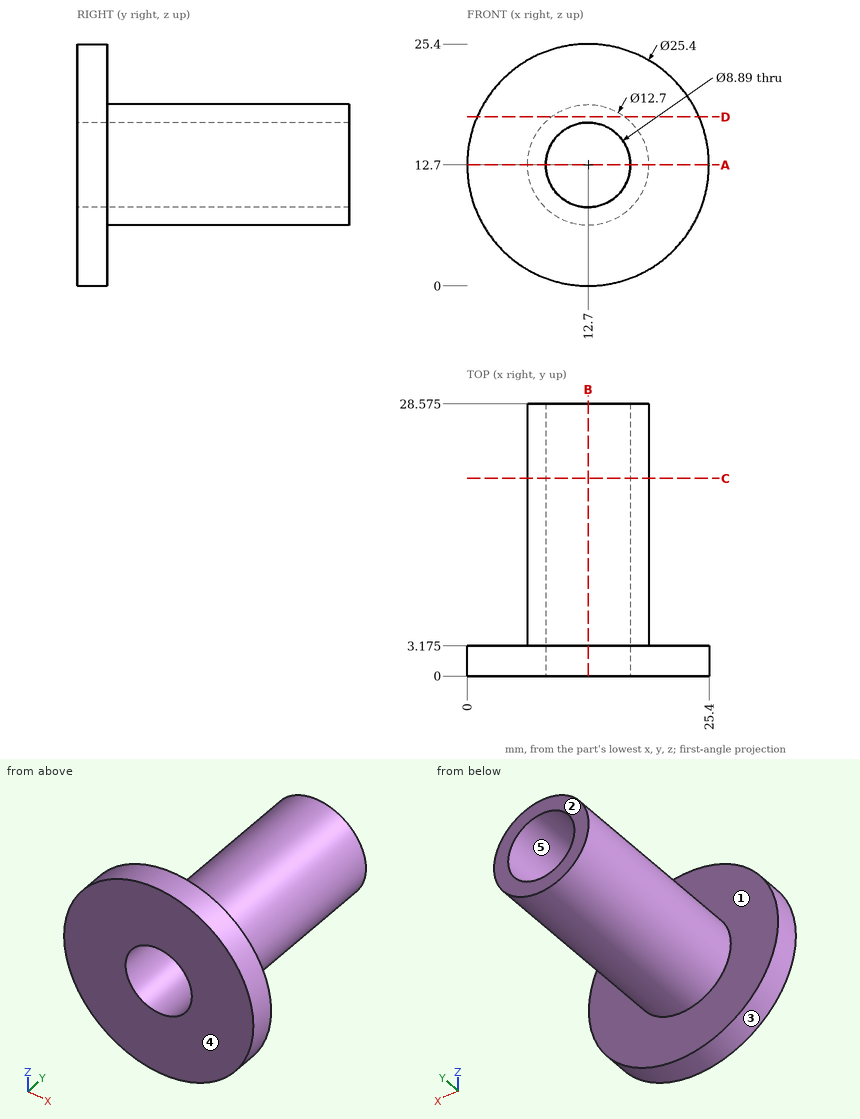
Print and shaded views of the part. All mm, measured from the part's lowest x, y and z. A direction names the side the tool comes from. Give positions to 0.01 mm unless a question says otherwise; leave off trailing zeros. Loops run counter-clockwise (first coordinate to the right, second up) from the corner with the lowest first, then second, coordinate; pieces in that order, holes last. Notation, with made-up numbers: (20.5, 1) -> (52.5, 1) arc R8 ccw to (52.5, 11) -> close; hole circle Ø9 at (-3.5, -9). An arc over 180 degrees is marked (long way). Answer in a Markdown table with one row per item.
Item 1: Tool access for the marked faces 1 and 2: list every direction of +Z, -Z, +X, -X, +Y, -Y with a clear straight run to the whole face (end or side of a thin tool).
Findings below:
| item | result |
|---|---|
| face 1 | +Y |
| face 2 | +Z, -Z, +X, -X, +Y |
Item 2: Flat gauge pins, fed straight in: P1, Ø10, axis at y = 20.5, z = 16, coming from the -X side; P2, Ø3, axis at x = 7.5, z = 20.5, coming from the +Y side (3 decimals); P3, Ø1.5, axis at x = 18.5, y = 16.5, coming from the -Z side. Where does each tip first touch, or does it go through?
Findings below:
| item | result |
|---|---|
| P1 | stops at x = 6.35 |
| P2 | stops at y = 3.175 |
| P3 | stops at z = 8.85 |
Item 3: Slice it at B-B on x = 12.7. Write the cut outline in (y, z) (3 decimals), plus the area to 3 significant figures.
Findings below:
| item | result |
|---|---|
| outline | (0, 0) -> (3.175, 0) -> (3.175, 6.35) -> (28.575, 6.35) -> (28.575, 8.255) -> (0, 8.255) -> close; (0, 17.145) -> (28.575, 17.145) -> (28.575, 19.05) -> (3.175, 19.05) -> (3.175, 25.4) -> (0, 25.4) -> close |
| area | 149 mm² |
Item 4: Slice it at A-A on z = 12.7. Write the cut outline in (x, y) (3 decimals), plus the area to 3 significant figures.
Findings below:
| item | result |
|---|---|
| outline | (0, 0) -> (8.255, 0) -> (8.255, 28.575) -> (6.35, 28.575) -> (6.35, 3.175) -> (0, 3.175) -> close; (17.145, 0) -> (25.4, 0) -> (25.4, 3.175) -> (19.05, 3.175) -> (19.05, 28.575) -> (17.145, 28.575) -> close |
| area | 149 mm² |
Item 5: Slice it at C-C on y = 20.75. Write the cut outline in (x, z) (3 decimals).
Findings below:
| item | result |
|---|---|
| outline | circle Ø12.7 at (12.7, 12.7); hole circle Ø8.89 at (12.7, 12.7) |
Item 6: Slice it at D-D on z = 17.75. Write the cut outline in (x, y) (3 decimals), plus the area to 3 significant figures.
Findings below:
| item | result |
|---|---|
| outline | (1.047, 0) -> (24.353, 0) -> (24.353, 3.175) -> (16.55, 3.175) -> (16.55, 28.575) -> (8.85, 28.575) -> (8.85, 3.175) -> (1.047, 3.175) -> close |
| area | 270 mm² |
Item 7: Probe line 1 along Z through (x, y) = (12.7, 22) (3 decimals); line 2 along Y through (x, z) = (1.5, 18.25) (3 decimals); line 3 along X through (y, z) = (23.5, 13.5). List the from-to ranges inside material, lowest first. Write a range as [from, to].
Findings below:
| item | result |
|---|---|
| line 1 | z = [6.35, 8.255], [17.145, 19.05] |
| line 2 | y = [0, 3.175] |
| line 3 | x = [6.4, 8.33], [17.07, 19] |
Item 8: Mould opens along Z. For the marked faces 3, 4 and 5 say: pulls with the +Z half, pulls with the -Z half, needs draft (parallel to the pull), parting line crosses it, or undercut.
Findings below:
| item | result |
|---|---|
| face 3 | parting line crosses it |
| face 4 | needs draft |
| face 5 | undercut |
